Autodesk Fusion 360 part; units mm, degrees
sketch "Unsorted Smarties Holder" plane through (0, 0, 0) normal (1, 0, 0) x (0, 1, 0)
  line L0 (0, 0) -> (93.3717, 0)
  line L1 (93.3717, 0) -> (93.3717, 143.115)
  line L2 (93.3717, 143.115) -> (45.2924, 143.115)
  line L3 (45.2924, 143.115) -> (-27.6283, 0)
  line L4 (-27.6283, 0) -> (0, 0)
  line L5 (-27.6283, 0) -> (93.3717, 0)
  line L6 (93.3717, 0) -> (93.3717, -6)
  line L7 (93.3717, -6) -> (-27.6283, -6)
  line L8 (-27.6283, -6) -> (-27.6283, 0)
  dimension "d5" = 143.115
  dimension "d14" = 63
  dimension "d23" = 121
  dimension "d31" = 6
extrude "Extrude1" add sketch "Unsorted Smarties Holder" along normal blind 270
sketch "Sketch3" plane through (270, 0, 0) normal (1, 0, 0) x (0, 1, 0)
  line L0 (93.3717, -6) -> (93.3717, 143.115)
  line L1 (93.3717, 143.115) -> (45.2924, 143.115)
  line L2 (45.2924, 143.115) -> (-27.6283, 0)
  line L3 (87.3717, 137.115) -> (87.3717, 0)
  line L4 (87.3717, 0) -> (-20.8944, 0)
  line L5 (-20.8944, 0) -> (48.9692, 137.115)
  line L6 (48.9692, 137.115) -> (87.3717, 137.115)
  line L7 (-27.6283, 0) -> (-27.6283, -6)
  line L8 (-27.6283, -6) -> (93.3717, -6)
  line L9 (-20.8944, 0) -> (87.3717, 0)
  line L10 (87.3717, 0) -> (87.3717, -6)
  line L11 (87.3717, -6) -> (-20.8944, -6)
  line L12 (-20.8944, -6) -> (-20.8944, 0)
  dimension "d15" = 6
  dimension "d16" = 6
  dimension "d17" = 6
  dimension "d18" = 6
  dimension "d32" = 6
  dimension "d33" = 6
extrude "Extrude3" cut sketch "Sketch3" against normal blind 258 from surface at -6 contours L4 L8 L9 L10 L11 L12 | L3 L4 L5 L6 L9
sketch "Smarties Feed" plane through (0, 93.3717, 0) normal (0, 1, 0) x (-1, 0, 0)
  line L0 (0, -6) -> (0, 143.115)
  line L1 (0, 143.115) -> (-270, 143.115)
  line L2 (-270, 143.115) -> (-270, -6)
  line L3 (-180, 108.115) -> (-90, 108.115)
  line L4 (-90, 108.115) -> (-90, 78.115)
  line L5 (-90, 78.115) -> (-180, 78.115)
  line L6 (-180, 78.115) -> (-180, 108.115)
  line L7 (-270, -6) -> (0, -6)
  dimension "d24" = 30
  dimension "d25" = 90
  dimension "d26" = 90
  dimension "d27" = 90
  dimension "d28" = 35
extrude "Extrude4" cut sketch "Smarties Feed" against normal blind 6 contours L3 L4 L5 L6
equation "polycarbonateThickness = 6 mm"
equation "d14 = 180 deg - 117 deg"
equation "d15 = polycarbonateThickness"
equation "d16 = polycarbonateThickness"
equation "d17 = polycarbonateThickness"
equation "d18 = polycarbonateThickness"
equation "d21 = -( 270 mm - 2 * polycarbonateThickness )"
equation "d28 = 41 mm - 6 mm"
Design review of the part built by this model. Coordinates are the model's own, in mm. A direction names the side the tool comes from. Coordinates: 2 decimals unless noted, no trailing zeros. Write each loop counter-clockwise with the first axis right and the second up, starting at its lowest first coordinate (ties: lowest second). Pieces come first, ordered by that corner, then holes.
1) Insertion check: pin 1 (10 mm diameter, centred on x = 34, y = 51, fed in from -Z); pin 2 (5 mm diameter, centred on x = 40, z = 99, fed in from -Y); pin 3 (5 mm diameter, centred on x = 122, y = 17.5, fed in from -Z). Each pin has a flat end and moves straight along its axis. Give the tip position at first contact, or say it passes through.
2) To check wall thickness, follow L1, parallel to X at y = 69.5, z = 37.5; L2, parallel to Z at x = 61, y = 58.5 (3 decimals); L3, parallel to Y at x = 103, z = 27. State the ranges of each line that lie inside material, in increasing order.
3) Add section D-D (x = 234). Write out the cut boundary in (y, z) (3 decimals), plus the area to 3 significant figures.
4) Add section A-A (x = 173.5). Write out the cut boundary in (y, z) (3 decimals), plus the area to 3 significant figures.
5) Machinability: for faces 4 (the flat face through (133, 93.372, 68)), 5 (the flat face through (137, 68, 137.115)), 6 (the flat face through (180, 90, 93)), which of the approach directions +Z, -Z, +X, -X, +Y, -Y give a long, thin tool a straight path to every point of the face, cutting with its end or side? Answer none if there is none.
6) Mouldability with a two-part tool opening along Z and no side actions: class faces 1 (the flat face through (136, 90, 108.115)), 2 (the flat face through (137, -20.894, -3)), 3 (the flat face through (133, 70, 143.115)) as +Z half, -Z half, draft (parallel to the pull), parting line (faces both ways), or undercut.
7) Add section C-C (z = 122.5). Write out the cut boundary in (x, y).
8) Add section B-B (y = 64). Write out the cut boundary in (x, z) (3 decimals).
Check result:
1. pin 1: stops at z = 131.29
1. pin 2: stops at y = 21.54
1. pin 3: stops at z = 70.45
2. L1: x = 0 to 6, 264 to 270
2. L2: z = 137.115 to 143.115
2. L3: y = -13.87 to -7.14, 87.37 to 93.37
3. outline: (-27.628, -6) - (-20.894, -6) - (-20.894, 0) - (48.969, 137.115) - (87.372, 137.115) - (87.372, -6) - (93.372, -6) - (93.372, 143.115) - (45.292, 143.115) - (-27.628, 0) - close
3. area: 2,120 mm2
4. outline: (-27.628, -6) - (-20.894, -6) - (-20.894, 0) - (48.969, 137.115) - (87.372, 137.115) - (87.372, 108.115) - (93.372, 108.115) - (93.372, 143.115) - (45.292, 143.115) - (-27.628, 0) - close; (87.372, -6) - (93.372, -6) - (93.372, 78.115) - (87.372, 78.115) - close
4. area: 1,940 mm2
5. face 4: +Z, -Z, +X, -X, +Y
5. face 5: -Z
5. face 6: +Y
6. face 1: undercut
6. face 2: draft
6. face 3: +Z half
7. outline: (0, 34.79) - (270, 34.79) - (270, 93.37) - (0, 93.37) - close; hole (6, 41.52) - (264, 41.52) - (264, 87.37) - (6, 87.37) - close
8. outline: (0, -6) - (6, -6) - (6, 137.115) - (264, 137.115) - (264, -6) - (270, -6) - (270, 143.115) - (0, 143.115) - close
